```python
from build123d import *

# Parameters (mm, degrees)
SKETCH1_W          = 107.95
SKETCH1_H          = 101.6
SKETCH1_R          = 40.5003
EXTRUDE1_DEPTH     = 57.15
CUT_EXTRUDE1_DEPTH = 108.95
SKETCH3_R          = 42.926
CUT_EXTRUDE2_DEPTH = 41.275
FILLET1_R          = 1.524
HOLE1_D            = 7.1374
HOLE1_DEPTH        = 101.6


with BuildPart() as part:
    # Sketch1 → Extrude1 (new body)
    with BuildSketch(Plane.XY):
        with Locations((0, 50.8)):
            Rectangle(SKETCH1_W, SKETCH1_H)
        with Locations((0, 50.8)):
            Circle(SKETCH1_R, mode=Mode.SUBTRACT)
    extrude(amount=-EXTRUDE1_DEPTH)

    # Sketch2 → Cut-Extrude1 (cut, through all)
    with BuildSketch(Plane(origin=(53.975, 0, 0), x_dir=(0, 0, -1), z_dir=(1, 0, 0))):
        Polygon((19.05, 101.6), (57.15, 35.56), (57.15, 101.6), align=None)
    extrude(amount=-CUT_EXTRUDE1_DEPTH, mode=Mode.SUBTRACT)

    # Sketch3 → Cut-Extrude2 (cut)
    with BuildSketch(Plane(origin=(0, 0, -57.15), x_dir=(-1, 0, 0), z_dir=(0, 0, -1))):
        with Locations(Location((0, 50.8, 0), (0, 0, 339.204742364))):  # turned: the seam where the file's is
            Circle(SKETCH3_R)
    extrude(amount=-CUT_EXTRUDE2_DEPTH, mode=Mode.SUBTRACT)

    # Fillet1
    fillet1_edges = [part.edges().sort_by_distance(p)[0] for p in [
        (40.129588535, 66.04, -15.875),
    ]]
    fillet(fillet1_edges, radius=FILLET1_R)

    # Hole1
    with Locations(Plane(origin=(0, 101.6, 0), x_dir=(-1, 0, 0), z_dir=(0, 1, 0))):
        with Locations((46.0502, -7.874), (-46.0248, -7.874)):
            Hole(HOLE1_D / 2, depth=HOLE1_DEPTH)


solid = part.part
```
Read the model definition and answer for the solid it produces. Units are mm, in the model's axes. A direction names the side the tool comes from. Give positions to 0.01 mm unless a question says otherwise; leave off trailing zeros. Order: outer loops, then holes, each group sorted by start corner. A loop starts at its lowest first (then second) coordinate and runs counter-clockwise, first axis right, second up. Notation, with made-up numbers: (29.5, -10.5) -> (57.5, -10.5) arc R17 ccw to (57.5, 19.5) -> close; hole circle Ø11 at (0, 41.5). An arc over 180 degrees is marked (long way). One line per item, written item: value. Start each with the question number.
(1) The part is cut by section B-B (x = 46.5). Determine the outline of the cut face in (y, z), and give its area (3 significant figures).
(2) The part is cut by section C-C (z = -29.5). Determine the outline of the cut face in (x, y) (3 decimals), and give its area (3 significant figures).
(3) The part is cut by section D-D (y = 28.5). State how many separate pieces and enclosed holes the cut face has, and give its area (3 significant figures).
(4) A tool of negligible diameter and unlimited length cuts with its end or side. For faces 4 (the flat face through (-1, 101.6, -9)), 5 (the cylindrical face through (-4.997, 8.166, -33.136)), from which of +Z, -Z, +X, -X, +Y, -Y can it reach the whole face along a straight path? Write none if from no direction.
(5) Flat-ended cylindrical pins translate along their axes: P1, Ø5, axis at x = -39, y = 39.5, coming from the -Z side; P2, Ø4, axis at x = -41.5, z = -45, coming from the -Y side; P3, Ø6.5, axis at x = 46.02, z = -7.87, coming from the -Y side. Find the tip coordinate at first contact, or state that the pin passes through.
(6) The part is cut by section A-A (y = 50.8). Determine the outline of the cut face in (x, z) (1 decimal).
(7) Straight lines are drawn through the part: L1, parallel to X at y = 50.5, z = -11 (3 decimals); L2, parallel to Y at x = 0, z = -41; L3, parallel to X at y = 45, z = -9 (3 decimals). For each, find the intervals that lie inside material, in ascending order.
(8) For a pull along X with two mould halves and no side action, classify faces 1 (the flat face through (-53.975, 39, -22)), 2 (the cylindrical face through (-42.646, 50.089, -6.802)), 3 (the flat face through (0.76, 98.39, -20.9)) as released by +X, released by -X, zero draft, split by the parting line, or undercut.
Taken from the geometry:
1. outline: (0, -57.15) -> (35.56, -57.15) -> (101.6, -19.05) -> (101.6, -11.41) -> (0, -11.41) -> close; (0, -4.34) -> (101.6, -4.34) -> (101.6, 0) -> (0, 0) -> close
1. area: 3,830 mm^2
2. outline: (-53.975, 0) -> (53.975, 0) -> (53.975, 83.487) -> (27.825, 83.487) arc R42.926 cw (long way) to (-27.825, 83.487) -> (-53.975, 83.487) -> close
2. area: 3,610 mm^2
3. separate pieces: 2
3. enclosed holes: 2
3. area: 1,990 mm^2
4. face 4: +Z, -Z, +X, -X, +Y
4. face 5: -Z
5. P1: z = -55.78
5. P2: y = 0
5. P3: through
6. outline: (-54, -48.4) -> (-42.9, -48.4) -> (-42.9, -17.4) arc R1.5 cw to (-41.4, -15.9) -> (-40.5, -15.9) -> (-40.5, 0) -> (-54, 0) -> close; (40.5, -15.9) -> (41.4, -15.9) arc R1.5 cw to (42.9, -17.4) -> (42.9, -48.4) -> (54, -48.4) -> (54, 0) -> (40.5, 0) -> close; hole circle Ø7.1 at (-46.1, -7.9); hole circle Ø7.1 at (46, -7.9)
7. L1: -53.975 to -47.772, -44.329 to -40.499, 40.499 to 44.303, 47.746 to 53.975
7. L2: 0 to 7.87
7. L3: -53.975 to -49.437, -42.664 to -40.083, 40.083 to 42.638, 49.411 to 53.975
8. face 1: released by -X
8. face 2: undercut
8. face 3: zero draft
